from build123d import *

# Parameters (mm, degrees)
SKETCH1_R           = 11.1125
SKETCH1_R_2         = 4.191
BASE_EXTRUDE_DEPTH  = 2.286
CUT_EXTRUDE1_DEPTH  = 16.880840925
BOSS_EXTRUDE1_DEPTH = 1.524
FILLET1_R           = 2.286


with BuildPart() as part:
    # Sketch1 → Base-Extrude (new body)
    with BuildSketch(Plane(origin=(0, 0, 0), x_dir=(-1, 0, 0), z_dir=(0, 1, 0))):
        with Locations(Location((0, 0, 0), (0, 0, 90))):
            Circle(SKETCH1_R)
        with Locations(Location((0, 0, 0), (0, 0, 90))):
            Circle(SKETCH1_R_2, mode=Mode.SUBTRACT)
    extrude(amount=BASE_EXTRUDE_DEPTH)

    # Sketch2 → Cut-Extrude1 (cut, through all)
    with BuildSketch(Plane(origin=(0, 2.286, 0), x_dir=(-1, 0, 0), z_dir=(0, 1, 0))):
        with BuildLine():
            Line((9.398, 5.930029701), (9.398, -5.930029701))
            ThreePointArc((9.398, -5.930029701), (11.1125, 0), (9.398, 5.930029701))
        make_face()
        with BuildLine():
            ThreePointArc((-9.398, 5.930029701), (-11.1125, 0), (-9.398, -5.930029701))
            Line((-9.398, -5.930029701), (-9.398, 5.930029701))
        make_face()
    extrude(amount=-CUT_EXTRUDE1_DEPTH, mode=Mode.SUBTRACT)

    # Sketch3 → Boss-Extrude1 (add)
    with BuildSketch(Plane(origin=(0, 2.286, 0), x_dir=(-1, 0, 0), z_dir=(0, 1, 0))):
        with BuildLine():
            Line((8.001, -7.711786774), (8.001, 7.711786774))
            ThreePointArc((8.001, 7.711786774), (8.744996559, 6.856580156), (9.398, 5.930029701))
            Line((9.398, 5.930029701), (9.398, -5.930029701))
            ThreePointArc((9.398, -5.930029701), (8.744996559, -6.856580156), (8.001, -7.711786774))
        make_face()
        with BuildLine():
            Line((-8.001, 7.711786774), (-8.001, -7.711786774))
            ThreePointArc((-8.001, -7.711786774), (-8.744996559, -6.856580156), (-9.398, -5.930029701))
            Line((-9.398, -5.930029701), (-9.398, 5.930029701))
            ThreePointArc((-9.398, 5.930029701), (-8.744996559, 6.856580156), (-8.001, 7.711786774))
        make_face()
    extrude(amount=BOSS_EXTRUDE1_DEPTH)

    # Fillet1
    fillet1_edges = [part.edges().sort_by_distance(p)[0] for p in [
        (9.398, 0, 0),
        (-9.398, 0, 0),
    ]]
    fillet(fillet1_edges, radius=FILLET1_R - 0.0001)  # a hair under: the kernel refuses the full size


solid = part.part
Work out the finished part from the listing and answer in its coordinate system (mm). A direction names the side the tool comes from. Round coordinates to 2 decimals unless told otherwise and drop trailing zeros. Write each loop counter-clockwise with the first axis right and the second up, starting at its lowest first coordinate (ties: lowest second). Pieces come first, ordered by that corner, then holes.
1) Given pin 1 Ø8 at (x, z) = (-0.5, 1) entering from +Y; pin 2 Ø1 at (y, z) = (0.5, 3) entering from -X; pin 3 Ø1.5 at (y, z) = (2, 7.5) entering from +X; pin 4 Ø2 at (y, z) = (2, 0) entering from -X, each flat-ended and moving along its own axis, determine where each tip first touches the part or whether it passes through.
2) Straight lines are drawn through the part: line 1 (X direction, y = 0.5, z = 0); line 2 (Y direction, x = 2.25, z = 5.75); line 3 (X direction, y = 1.65, z = 0). For each, find the intervals that lie inside material, in ascending order.
3) A cutting plane is placed at D-D (y = 2.05). Give the vertices of the cut face in (x, z) (1 decimal), plus the area to 3 significant figures.
4) A cutting plane is placed at C-C (z = 0). Give the vertices of the cut face in (x, y), plus the area to 3 significant figures.
5) A tool of negligible diameter and unlimited length cuts with its end or side. For faces 1 (the flat face through (-9, 3.81, 0)), 2 (the flat face through (8.001, 3, 0)), from which of +Z, -Z, +X, -X, +Y, -Y can it reach the whole face along a straight path? Write none if from no direction.
6) The mould has two halves that part along X. Classify faces 3 (the flat face through (4, 2.286, 2)), 4 (the flat face through (-5, 0, 0)), 5 (the flat face through (-8.001, 3, 0)), 6 (the cylindrical face through (9, 1, 0)): pulls with the +X half, pulls with the -X half, needs draft (parallel to the pull), parting line crosses it, or undercut.
7) A cutting plane is placed at A-A (y = 3.5). Give the vertices of the cut face in (x, z) (1 decimal), plus the area to 3 significant figures.
8) A cutting plane is placed at B-B (x = 0). Give the vertices of the cut face in (y, z).
Completed:
1. pin 1: stops at y = 2.29
1. pin 2: stops at x = -9
1. pin 3: stops at x = 8.83
1. pin 4: stops at x = -9.4
2. line 1: x = -8.54 to -4.19, 4.19 to 8.54
2. line 2: y = 0 to 2.29
2. line 3: x = -9.31 to -4.19, 4.19 to 9.31
3. outline: (-9.4, -5.9) arc R11.1 ccw to (9.4, -5.9) - (9.4, 5.9) arc R11.1 ccw to (-9.4, 5.9) - close; hole circle Ø8.4 at (0, 0)
3. area: 305 mm2
4. outline: (-9.4, 2.29) arc R2.29 ccw to (-7.11, 0) - (-4.19, 0) - (-4.19, 2.29) - (-8, 2.29) - (-8, 3.81) - (-9.4, 3.81) - close; (4.19, 0) - (7.11, 0) arc R2.29 ccw to (9.4, 2.29) - (9.4, 3.81) - (8, 3.81) - (8, 2.29) - (4.19, 2.29) - close
4. area: 25.8 mm2
5. face 1: +Z, -Z, +X, -X, +Y
5. face 2: +Z, -Z, +Y
6. face 3: undercut
6. face 4: needs draft
6. face 5: undercut
6. face 6: pulls with the +X half
7. outline: (-9.4, -5.9) arc R11.1 ccw to (-8, -7.7) - (-8, 7.7) arc R11.1 ccw to (-9.4, 5.9) - close; (8, -7.7) arc R11.1 ccw to (9.4, -5.9) - (9.4, 5.9) arc R11.1 ccw to (8, 7.7) - close
7. area: 38.5 mm2
8. outline: (0, -11.11) - (2.29, -11.11) - (2.29, -4.19) - (0, -4.19) - close; (0, 4.19) - (2.29, 4.19) - (2.29, 11.11) - (0, 11.11) - close
